Autodesk Inventor part; units mm, degrees
ref_plane "YZ Plane" through (0, 0, 0) normal (1, 0, 0) x (0, 1, 0)
ref_plane "XZ Plane" through (0, 0, 0) normal (0, 1, 0) x (-1, 0, 0)
ref_plane "XY Plane" through (0, 0, 0) normal (0, 0, 1) x (1, 0, 0)
sketch "Sketch1" plane through (0, 0, 0) normal (0, 0, 1) x (1, 0, 0)
  line L0 (262.89, 253.3796) -> (525.78, 101.6)
  line L1 (525.78, 101.6) -> (525.78, -201.9592) construction
  line L2 (525.78, -201.9592) -> (262.89, -353.7388) construction
  line L3 (262.89, -353.7388) -> (0, -201.9592) construction
  line L4 (0, -201.9592) -> (0, 101.6) construction
  line L5 (0, 101.6) -> (262.89, 253.3796)
  line L6 (0, 101.6) -> (0, 0)
  line L7 (0, 0) -> (525.78, 0)
  line L8 (525.78, 0) -> (525.78, 101.6)
  point P0 (262.89, -50.1796)
  dimension "d0" = 525.78
  dimension "d1" = 101.6
extrude "Extrusion1" add sketch "Sketch1" along normal blind 25.4
sketch "Sketch2" plane through (0, 0, 25.4) normal (0, 0, 1) x (1, 0, 0)
  circle A0 centre (262.89, 121.3796) radius 60
  line L0 (0, 0) -> (525.78, 0)
  point P0 (262.89, 0)
  dimension "d4" = 121.3796
  dimension "d5" = 120
extrude "Extrusion2" cut sketch "Sketch2" against normal through all
sketch "Sketch3" plane through (0, 0, 25.4) normal (0, 0, 1) x (1, 0, 0)
  circle A0 centre (262.89, 121.3796) radius 60 construction
  line L0 (0, 101.6) -> (0, 0) construction
  line L1 (0, 0) -> (525.78, 0) construction
  line L2 (525.78, 0) -> (525.78, 101.6) construction
  line L3 (525.78, 101.6) -> (262.89, 253.3796) construction
  line L4 (262.89, 253.3796) -> (0, 101.6) construction
  line L5 (12.7, 94.2677) -> (12.7, 12.7) construction
  line L6 (12.7, 12.7) -> (513.08, 12.7) construction
  line L7 (513.08, 12.7) -> (513.08, 94.2677) construction
  line L8 (513.08, 94.2677) -> (262.89, 238.7149) construction
  line L9 (262.89, 238.7149) -> (12.7, 94.2677) construction
  circle A1 centre (12.7, 88.5) radius 2
  circle A2 centre (12.7, 38.5) radius 2
  line L10 (12.7, 88.5) -> (12.7, 38.5) construction
  circle A3 centre (51.1925, 116.4913) radius 2
  circle A4 centre (224.3975, 216.4913) radius 2
  circle A5 centre (137.795, 166.4913) radius 2
  circle A6 centre (51.1925, 12.7) radius 2
  circle A7 centre (137.795, 12.7) radius 2
  circle A8 centre (224.3975, 12.7) radius 2
  circle A9 centre (262.89, 12.7) radius 2
  line L11 (51.1925, 116.4913) -> (224.3975, 216.4913) construction
  line L12 (262.89, 238.7149) -> (262.89, 253.3796)
  line L13 (525.78, 101.6) -> (525.78, 0) construction
  line L14 (513.08, 94.2677) -> (513.08, 12.7) construction
  circle A10 centre (513.08, 88.5) radius 2
  circle A11 centre (513.08, 38.5) radius 2
  line L15 (513.08, 88.5) -> (513.08, 38.5) construction
  circle A12 centre (474.5875, 116.4913) radius 2
  circle A13 centre (301.3825, 216.4913) radius 2
  circle A14 centre (387.985, 166.4913) radius 2
  circle A15 centre (474.5875, 12.7) radius 2
  circle A16 centre (387.985, 12.7) radius 2
  circle A17 centre (301.3825, 12.7) radius 2
  circle A18 centre (262.89, 12.7) radius 2
  line L16 (474.5875, 116.4913) -> (301.3825, 216.4913) construction
  line L17 (30.0651, 0) -> (30.0651, 25.4)
  line L18 (30.0651, 25.4) -> (30.0651, 101.6)
  point P0 (525.78, 0)
  point P1 (30.0651, 63.5)
  point P2 (12.7, 63.5)
  dimension "d8" = 12.7
  dimension "d9" = 4
  dimension "d10" = 4
  dimension "d11" = 50
  dimension "d12" = 4
  dimension "d13" = 4
  dimension "d14" = 4
  dimension "d15" = 4
  dimension "d16" = 4
  dimension "d17" = 4
  dimension "d18" = 4
  dimension "d19" = 200
  dimension "d38" = 25.4
extrude "Extrusion3" cut sketch "Sketch3" against normal through all contours A1 | A2 | A3 | A4 | A7 | A8 | A10 | A11 | A12 | A13 | A16 | A17
sketch "Sketch5" plane through (0, 0, 0) normal (0, 0, -1) x (-1, 0, 0)
  circle A0 centre (-513.08, 88.5) radius 2
  circle A1 centre (-387.985, 12.7) radius 2
  circle A2 centre (-224.3975, 216.4913) radius 2
  circle A3 centre (-12.7, 38.5) radius 2
  circle A4 centre (-12.7, 88.5) radius 2
  circle A5 centre (-51.1925, 116.4913) radius 2
  circle A6 centre (-137.795, 12.7) radius 2
  circle A7 centre (-301.3825, 216.4913) radius 2
  circle A8 centre (-474.5875, 116.4913) radius 2
  circle A9 centre (-513.08, 38.5) radius 2
  circle A10 centre (-262.89, 121.3796) radius 60
  line L0 (0, 0) -> (0, 101.6)
  line L1 (0, 101.6) -> (-262.89, 253.3796)
  line L2 (-262.89, 253.3796) -> (-525.78, 101.6)
  line L3 (-525.78, 101.6) -> (-525.78, 0)
  line L4 (-525.78, 0) -> (0, 0)
  line L5 (-25.4, 25.4) -> (-25.4, 86.9353)
  line L6 (-25.4, 86.9353) -> (-262.89, 224.0502)
  line L7 (-262.89, 224.0502) -> (-500.38, 86.9353)
  line L8 (-500.38, 86.9353) -> (-500.38, 25.4)
  line L9 (-500.38, 25.4) -> (-25.4, 25.4)
  circle A11 centre (-262.89, 121.3796) radius 85.4
  dimension "d26" = 25.4
  dimension "d27" = 25.4
extrude "Extrusion5" cut sketch "Sketch5" against normal blind 19.05 contours L9 L8 L7 L6 L5
sketch "Sketch6" plane through (0, 0, 25.4) normal (0, 0, 1) x (1, 0, 0)
  circle A0 centre (513.08, 38.5) radius 2 construction
  circle A1 centre (513.08, 88.5) radius 2 construction
  circle A2 centre (387.985, 12.7) radius 2 construction
  circle A3 centre (224.3975, 216.4913) radius 2 construction
  circle A4 centre (12.7, 38.5) radius 2 construction
  circle A5 centre (12.7, 88.5) radius 2 construction
  circle A6 centre (51.1925, 116.4913) radius 2 construction
  circle A7 centre (137.795, 12.7) radius 2 construction
  circle A8 centre (301.3825, 216.4913) radius 2 construction
  circle A9 centre (474.5875, 116.4913) radius 2 construction
  circle A10 centre (513.08, 38.5) radius 2 construction
  circle A11 centre (262.89, 121.3796) radius 60 construction
  line L0 (0, 101.6) -> (0, 0) construction
  line L1 (0, 0) -> (525.78, 0) construction
  line L2 (525.78, 0) -> (525.78, 101.6) construction
  line L3 (525.78, 101.6) -> (262.89, 253.3796) construction
  line L4 (262.89, 253.3796) -> (0, 101.6) construction
  circle A12 centre (513.08, 38.5) radius 2
  circle A13 centre (513.08, 38.5) radius 6.5
  circle A14 centre (513.08, 88.5) radius 2
  circle A15 centre (513.08, 88.5) radius 6.5
  circle A16 centre (474.5875, 116.4913) radius 2
  circle A17 centre (474.5875, 116.4913) radius 6.5
  circle A18 centre (301.3825, 216.4913) radius 2
  circle A19 centre (301.3825, 216.4913) radius 6.5
  circle A20 centre (387.985, 12.7) radius 2
  circle A21 centre (387.985, 12.7) radius 6.5
  line L5 (262.89, 253.3796) -> (262.89, 364.4597)
  circle A22 centre (12.7, 88.5) radius 2 construction
  circle A23 centre (12.7, 38.5) radius 6.5
  circle A24 centre (12.7, 88.5) radius 6.5
  circle A25 centre (51.1925, 116.4913) radius 6.5
  circle A26 centre (224.3975, 216.4913) radius 6.5
  circle A27 centre (137.795, 12.7) radius 6.5
  circle A28 centre (224.3975, 12.7) radius 2
  circle A29 centre (301.3825, 12.7) radius 2
  circle A30 centre (224.3975, 12.7) radius 6.5
  circle A31 centre (301.3825, 12.7) radius 6.5
  dimension "d30" = 13
  dimension "d31" = 13
  dimension "d32" = 13
  dimension "d33" = 13
  dimension "d34" = 13
  dimension "d39" = 13
  dimension "d40" = 13
extrude "Extrusion6" cut sketch "Sketch6" against normal blind 12.7 contours A12 | A13 | A14 | A15 | A16 | A17 | A18 | A19 | A20 | A21 | A23 | A24 | A25 | A26 | A27 | A29 | A30 | A31
sketch "Sketch8" plane through (0, 0, 25.4) normal (0, 0, 1) x (1, 0, 0)
  circle A0 centre (50, 12.7) radius 2
  circle A1 centre (475.78, 12.7) radius 2
  line L0 (0, 101.6) -> (0, 0)
  line L1 (525.78, 0) -> (525.78, 101.6)
  circle A2 centre (387.985, 12.7) radius 2
  dimension "d41" = 4
  dimension "d42" = 4
  dimension "d43" = 50
  dimension "d44" = 50
extrude "Extrusion7" cut sketch "Sketch8" against normal through all
sketch "Sketch9" plane through (0, 0, 25.4) normal (0, 0, 1) x (1, 0, 0)
  circle A0 centre (50, 12.7) radius 2
  circle A1 centre (475.78, 12.7) radius 2
  circle A2 centre (50, 12.7) radius 6.5
  circle A3 centre (475.78, 12.7) radius 2
  circle A4 centre (475.78, 12.7) radius 6.5
  point P0 (0, 0)
  dimension "d47" = 13
  dimension "d48" = 13
extrude "Extrusion8" cut sketch "Sketch9" against normal blind 12.7 contours A0 | A1 | A2 | A4
properties part number "HB04" material "Polyethylene, High Density"
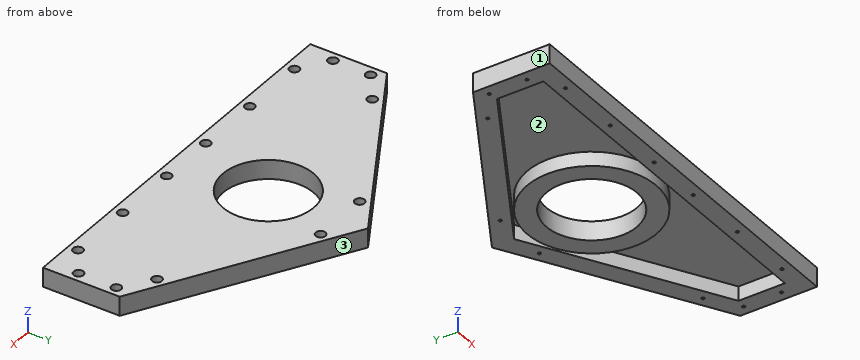
The model under review builds one solid part; all positions refer to its coordinate system, in mm. Face numbers are marked on the shaded views. Coordinates: 2 decimals unless noted, no trailing zeros. Loops run counter-clockwise (first coordinate to the right, second up) from the corner with the lowest first, then second, coordinate; pieces in that order, holes last.
(1) Consider section A-A, the plane z = 4.5. Give the number of separate pieces and of enclosed holes in the cut face, plus the area to 3 significant figures.
Determined:
separate pieces: 2
enclosed holes: 16
area: 43,000 mm2
(2) Insertion check: P1, Ø4, axis at x = 53.5, y = 116, coming from the +Z side; P2, Ø3, axis at y = 198.5, z = 6, coming from the +X side; P3, Ø1, axis at y = 115, z = 13.5, coming from the -X side. Each pin has a flat end and moves straight along its axis. Give the tip position at first contact, or say it passes through.
Determined:
P1: stops at z = 12.7
P2: stops at x = 360.54
P3: stops at x = 22.34
(3) Consider section C-C, the plane x = 341.5. Give the boundary of the cut face in (y, z), plus the area to 3 significant figures.
Determined:
outline: (0, 0) - (25.4, 0) - (25.4, 19.05) - (88.01, 19.05) - (88.01, 0) - (154.75, 0) - (154.75, 19.05) - (178.66, 19.05) - (178.66, 0) - (207.99, 0) - (207.99, 25.4) - (0, 25.4) - close
area: 3,630 mm2
(4) Draft analysis for pull direction Y (two halves, no side actions). For the marked faces 1, 2 and 3, state which applies: +Y half, -Y half, draft (parallel to the pull), parting line (faces both ways), or undercut.
Determined:
face 1: draft
face 2: undercut
face 3: +Y half
(5) Wall thickness on L1, parallel to Y at x = 263, z = 4.25; L2, parallel to X at y = 43.5, z = 13; L3, parallel to Y at x = 196.5, z = 13.75: over which ranges is each line inside the solid? List them lowest first.
Determined:
L1: y = 0 to 25.4, 35.98 to 61.38, 181.38 to 206.78, 223.99 to 253.32
L2: x = 0 to 8.55, 16.85 to 25.4, 227.85 to 297.93, 500.38 to 508.93, 517.23 to 525.78
L3: y = 0 to 25.4, 67.66 to 175.1, 185.72 to 215.05
(6) Consider section B-B, the plane y = 70.5. Give the boundary of the cut face in (x, z).
Determined:
outline: (0, 0) - (25.4, 0) - (25.4, 19.05) - (194.3, 19.05) - (194.3, 0) - (231.09, 0) - (231.09, 25.4) - (0, 25.4) - close; (294.69, 0) - (331.48, 0) - (331.48, 19.05) - (500.38, 19.05) - (500.38, 0) - (525.78, 0) - (525.78, 25.4) - (294.69, 25.4) - close
